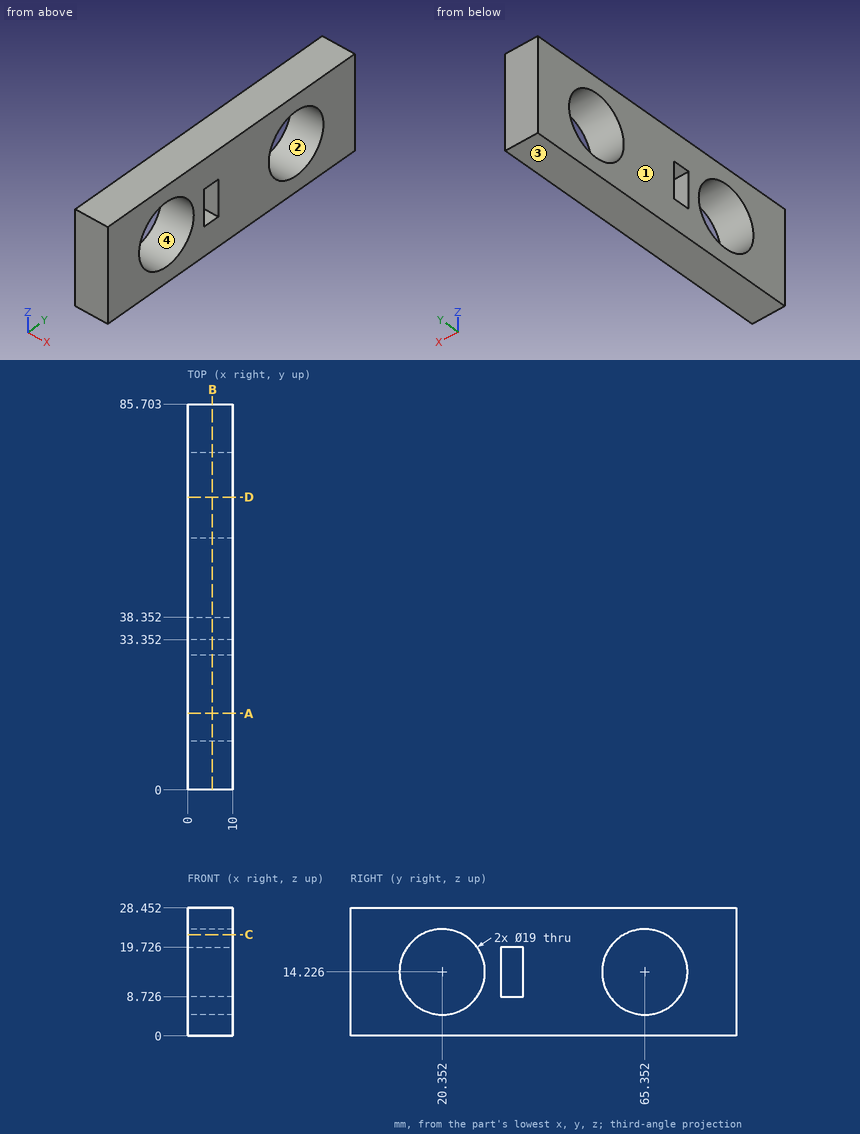
The figure shows three views and two pictorial views of one solid part (mm, origin at its lowest corner). Answer the questions. Give positions to 0.01 mm unless a question says otherwise; leave off trailing zeros. Write each loop counter-clockwise with the first axis right and the second up, starting at its lowest first coordinate (ties: lowest second). Pieces come first, ordered by that corner, then holes.
Q1. The part is cut by section D-D on y = 65. Give the vertices of the cut face in (x, z).
Answer:
outline: (0, 0) - (10, 0) - (10, 4.73) - (0, 4.73) - close; (0, 23.72) - (10, 23.72) - (10, 28.45) - (0, 28.45) - close
Q2. For a pull along Z with two mould halves and no side action, classify the marked faces 1, 2, 3 and 4 as released by +Z, released by -Z, zero draft, split by the parting line, or undercut.
Answer:
face 1: zero draft
face 2: undercut
face 3: released by -Z
face 4: undercut
Q3. The part is cut by section B-B on x = 5.5. Give the vertices of the cut face in (y, z).
Answer:
outline: (0, 0) - (85.7, 0) - (85.7, 28.45) - (0, 28.45) - close; hole circle Ø19 at (20.35, 14.23); hole (33.35, 8.73) - (38.35, 8.73) - (38.35, 19.73) - (33.35, 19.73) - close; hole circle Ø19 at (65.35, 14.23)
Q4. Given pin 1 (11.5 mm diameter, centred on y = 65.35, z = 14.23, fed in from -X), flat-ended and moving along its own axis, determine where the tip first touches the part or whether it passes through.
Answer:
pin 1: passes through
Q5. Straight lines are drawn through the part: L1, parallel to Y at x = 2.5, z = 14 (1 decimal); L2, parallel to Y at x = 7.75, z = 8.25 (1 decimal); L3, parallel to Y at x = 4.75, z = 20.5 (1 decimal). For each, find the intervals that lie inside material, in ascending order.
Answer:
L1: y = 0 to 10.9, 29.8 to 33.4, 38.4 to 55.9, 74.8 to 85.7
L2: y = 0 to 13, 27.7 to 58, 72.7 to 85.7
L3: y = 0 to 13.2, 27.5 to 58.2, 72.5 to 85.7
Q6. The part is cut by section C-C on z = 22.5. Give the vertices of the cut face in (x, y).
Answer:
outline: (0, 0) - (10, 0) - (10, 15.68) - (0, 15.68) - close; (0, 25.02) - (10, 25.02) - (10, 60.68) - (0, 60.68) - close; (0, 70.02) - (10, 70.02) - (10, 85.7) - (0, 85.7) - close
Q7. The part is cut by section A-A on y = 17. Give the vertices of the cut face in (x, z) (1 decimal), and give its area (3 significant figures).
Answer:
outline: (0, 0) - (10, 0) - (10, 5.3) - (0, 5.3) - close; (0, 23.1) - (10, 23.1) - (10, 28.5) - (0, 28.5) - close
area: 107 mm2
